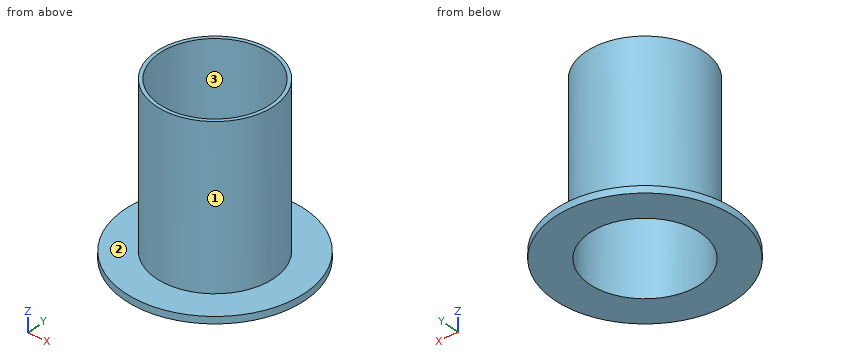
```python
from build123d import *

# Parameters (mm, degrees)
TUBE001_R     = 41.275
TUBE001_R_2   = 25.4
TUBE001_DEPTH = 3.175
TUBE_R        = 26.9875
TUBE_R_2      = 25.4
TUBE_DEPTH    = 76.2


with BuildPart() as tube001:
    # Tube001 → Tube001 (new body)
    with BuildSketch(Plane.XY):
        Circle(TUBE001_R)
        Circle(TUBE001_R_2, mode=Mode.SUBTRACT)
    extrude(amount=TUBE001_DEPTH)


with BuildPart() as fusion:
    # Tube → Tube (new body)
    with BuildSketch(Plane.XY):
        Circle(TUBE_R)
        Circle(TUBE_R_2, mode=Mode.SUBTRACT)
    extrude(amount=TUBE_DEPTH)

    # Fusion: union Tube001
    add(tube001.part)


solid = fusion.part
```
Input: part model. Units: mm. Frame: model coordinates. Face numbers are marked on the shaded views. Give positions to 0.01 mm unless a question says otherwise; leave off trailing zeros. Order: outer loops, then holes, each group sorted by start corner. A loop starts at its lowest first (then second) coordinate and runs counter-clockwise, first axis right, second up. Notation, with made-up numbers: M 81,30.25 L 121,30.25 A22 ccw 121,44.25 Z; hole C 84,26 d5. An arc over 180 degrees is marked long. Return JSON: item names as keys, results as strings.
Item 1: Cut plane D-D (x = 32). Return loops of the section in (y, z) (3 decimals).
Solutions:
{"outline": "M -26.07,0 L 26.07,0 L 26.07,3.175 L -26.07,3.175 Z"}
Item 2: First-contact query: P1, Ø8, axis at x = -33, z = 43.5, coming from the +Y side; P2, Ø2, axis at x = 20, z = 37, coming from the -Y side; P3, Ø4, axis at y = 5, z = 56, coming from the -X side; P4, Ø1.5, axis at x = -27.5, y = -19.5, coming from the +Z side (3 decimals). Flat tips, straight axial feed; report the tip coordinate or a pass-through.
Solutions:
{"P1": "through", "P2": "y = -19.17", "P3": "x = -26.82", "P4": "z = 3.175"}
Item 3: Ray query, probe 1 along Y at (x, z) = (0, 59); probe 2 along Z at (x, y) = (31.5, -22) (3 decimals); probe 3 along X at (y, z) = (-17.5, 37.5). Return the intervals inside material, ascending.
Solutions:
{"probe 1": "-26.99 to -25.4, 25.4 to 26.99", "probe 2": "0 to 3.175", "probe 3": "-20.54 to -18.41, 18.41 to 20.54"}
Item 4: Cut plane A-A (x = 0). Return loops of the section in (y, z) (1 decimal), then the cut area to 3 significant figures.
Solutions:
{"outline": "M -41.3,0 L -25.4,0 L -25.4,76.2 L -27,76.2 L -27,3.2 L -41.3,3.2 Z; M 25.4,0 L 41.3,0 L 41.3,3.2 L 27,3.2 L 27,76.2 L 25.4,76.2 Z", "area": "333 mm^2"}
Item 5: Pull-direction query (X, two-part tool) for the marked faces 1, 2 and 3; classes: +X half, -X half, draft (parallel to the pull), parting line (faces both ways), or undercut.
Solutions:
{"face 1": "parting line", "face 2": "draft", "face 3": "undercut"}
Item 6: Cut plane C-C (z = 56.5). Return loops of the section in (x, y) (1 decimal), then the cut area to 3 significant figures.
Solutions:
{"outline": "C 0,0 d54; hole C 0,0 d50.8", "area": "261 mm^2"}
